The listing builds one solid part. Answer for the finished solid, in the listing's coordinates (mm). A direction names the side the tool comes from. Give positions to 0.01 mm unless a question says otherwise; leave off trailing zeros. Write each loop counter-clockwise with the first axis right and the second up, starting at its lowest first coordinate (ties: lowest second). Pieces come first, ordered by that corner, then holes. Notation, with made-up numbers: (-8.5, 79) -> (38.5, 79) arc R22 ccw to (38.5, 97) -> close; hole circle Ø11 at (-33.5, -8.5). An arc over 180 degrees is marked (long way). Write each question's results on one line, items separated by ' | '. Start each with the question number.
Autodesk Inventor part; units mm, degrees
ref_plane "YZ Plane" through (0, 0, 0) normal (1, 0, 0) x (0, 1, 0)
ref_plane "XZ Plane" through (0, 0, 0) normal (0, 1, 0) x (-1, 0, 0)
ref_plane "XY Plane" through (0, 0, 0) normal (0, 0, 1) x (1, 0, 0)
sketch "Эскиз4" plane through (0, 0, 0) normal (0, 0, 1) x (1, 0, 0)
  line L0 (45.2395, 25.2453) -> (-44.981, 25.2453)
  line L1 (-44.981, 25.2453) -> (-44.981, -24.4084)
  line L2 (-44.981, -24.4084) -> (45.2395, -24.4084)
  line L3 (45.2395, -24.4084) -> (45.2395, 25.2453)
  point P0 (0, 0)
extrude "Прямоугольник_" add sketch "Эскиз4" along normal blind 15
sketch "Прямоугольник" plane through (0, 0, 0) normal (0, 0, 1) x (1, 0, 0)
  line L0 (-77.4921, 158.0418) -> (133.4103, 158.0418) construction
  line L1 (133.4103, 158.0418) -> (133.4103, -71.9132) construction
  line L2 (133.4103, -71.9132) -> (-77.4921, -71.9132) construction
  line L3 (-77.4921, -71.9132) -> (-77.4921, 158.0418) construction
  line L4 (44.9907, 25.2614) -> (-45.0093, 25.2614)
  line L5 (-45.0093, 25.2614) -> (-45.0093, -24.7386)
  line L6 (-45.0093, -24.7386) -> (44.9907, -24.7386)
  line L7 (44.9907, -24.7386) -> (44.9907, 25.2614)
  point P0 (0, 0)
  dimension "d17" = 90
  dimension "d20" = 50
sketch "Три отверстия по краям" plane through (0, 0, 15) normal (0, 0, 1) x (1, 0, 0)
  circle A0 centre (-34.9124, 0) radius 5
  circle A1 centre (35.035, 15.2594) radius 5
  circle A2 centre (35.035, -14.8643) radius 5
  point P0 (0, 0)
  dimension "d12" = 10
  dimension "d13" = 10
  dimension "d14" = 10
extrude "3 отверстия по краям" cut sketch "Три отверстия по краям" against normal blind 800
sketch "Возвышенность по центру" plane through (0, 0, 15) normal (0, 0, 1) x (1, 0, 0)
  circle A0 centre (0, 0) radius 15
  dimension "d21" = 30
extrude "Возвышенность" add sketch "Возвышенность по центру" along normal blind 25
sketch "Эскиз7" plane through (0, 0, 0) normal (0, 0, -1) x (-1, 0, 0)
  circle A0 centre (0, 0) radius 9
  dimension "d24" = 18
extrude "Внутренняя часть внутри возв" cut sketch "Эскиз7" against normal blind 38
sketch "Эскиз8" plane through (0, 0, 15) normal (0, 0, 1) x (1, 0, 0)
  circle A0 centre (0, 0) radius 15
  line L0 (45.2395, -24.4084) -> (45.2395, 25.2453)
  line L1 (-14.1421, 5) -> (-24.1421, 5)
  line L2 (-24.1421, 5) -> (-24.1421, -5)
  line L3 (-24.1421, -5) -> (-14.1421, -5)
  line L4 (14.1421, 5) -> (24.1421, 5)
  line L5 (24.1421, 5) -> (24.1421, -5)
  line L6 (24.1421, -5) -> (14.1421, -5)
  dimension "d27" = 10
  dimension "d28" = 10
  dimension "d29" = 10
extrude "Детали по бокам возв." add sketch "Эскиз8" along normal blind 20 contours A0 L4 L5 L6 | A0 L3 L2 L1
properties part number "Основание"
1. The mould has two halves that part along Y. Classify faces 6 (the flat face through (-1, -24.408, 7)), 7 (the cylindrical face through (-39.908, 0.22, 7.605)), 8 (the flat face through (24.142, 0, 25)): pulls with the +Y half, pulls with the -Y half, needs draft (parallel to the pull), parting line crosses it, or undercut.
2. A tool of negligible diameter and unlimited length cuts with its end or side. For faces 1 (the flat face through (19, -5, 25)), 2 (the flat face through (19, 5, 25)), 3 (the flat face through (-19, -5, 25)), 4 (the cylindrical face through (-3.252, 14.643, 27.325)), 5 (the flat face through (0, 0, 38)), from which of +Z, -Z, +X, -X, +Y, -Y can it reach the whole face along a straight path? Write none if from no direction.
3. Each of these flat-tipped pins is pushed along its axis until it touches: pin 1 Ø5 at (y, z) = (-2, 20.5) entering from -X; pin 2 Ø8 at (x, z) = (-27.5, 29) entering from -Y; pin 3 Ø11 at (x, z) = (-20.5, 21.5) entering from +Y; pin 4 Ø9 at (x, y) = (-34.91, 0) entering from -Z. Where does it stop, or does it pass through?
4. Section A-A (y = 0) is taken. Write down the section's boundary in (x, z), then the cut area to 3 significant figures.
5. Section B-B (x = 0) is taken. Write down the section's boundary in (y, z).
6. Section D-D (x = 31) is taken. Write down the section's boundary in (y, z), then the cut area to 3 significant figures.
7. Consider probe 1 along Z at (x, y) = (24, 3.5); probe 2 along Z at (x, y) = (23, -8.5); probe 3 along X at (y, z) = (-0.5, 31). Determine where each line is inside the solid, lowest interval first. Write a range as [from, to].
8. Section C-C (z = 8) is taken. Write down the section's boundary in (x, y) (1 decimal).
Results:
1) face 6: pulls with the -Y half | face 7: undercut | face 8: needs draft
2) face 1: +Z, +X, -Y | face 2: +Z, +X, +Y | face 3: +Z, -X, -Y | face 4: +Z | face 5: -Z
3) pin 1: stops at x = -24.14 | pin 2: stops at y = -5 | pin 3: stops at y = 5 | pin 4: passes through
4) outline: (-44.98, 0) -> (-39.91, 0) -> (-39.91, 15) -> (-44.98, 15) -> close; (-29.91, 0) -> (-9, 0) -> (-9, 38) -> (9, 38) -> (9, 0) -> (45.24, 0) -> (45.24, 15) -> (24.14, 15) -> (24.14, 35) -> (15, 35) -> (15, 40) -> (-15, 40) -> (-15, 35) -> (-24.14, 35) -> (-24.14, 15) -> (-29.91, 15) -> close | area: 1,630 mm²
5) outline: (-24.41, 0) -> (-9, 0) -> (-9, 38) -> (9, 38) -> (9, 0) -> (25.25, 0) -> (25.25, 15) -> (15, 15) -> (15, 40) -> (-15, 40) -> (-15, 15) -> (-24.41, 15) -> close
6) outline: (-24.41, 0) -> (-17.82, 0) -> (-17.82, 15) -> (-24.41, 15) -> close; (-11.91, 0) -> (12.31, 0) -> (12.31, 15) -> (-11.91, 15) -> close; (18.21, 0) -> (25.25, 0) -> (25.25, 15) -> (18.21, 15) -> close | area: 568 mm²
7) probe 1: z = [0, 35] | probe 2: z = [0, 15] | probe 3: x = [-24.14, -8.99], [8.99, 24.14]
8) outline: (-45, -24.4) -> (45.2, -24.4) -> (45.2, 25.2) -> (-45, 25.2) -> close; hole circle Ø10 at (-34.9, 0); hole circle Ø18 at (0, 0); hole circle Ø10 at (35, -14.9); hole circle Ø10 at (35, 15.3)
